For this review, take the finished solid that the model builds, in its own axes (mm). A direction names the side the tool comes from. Round coordinates to 2 decimals unless told otherwise and drop trailing zeros. Order: outer loops, then holes, each group sorted by start corner. A loop starts at its lowest first (then second) coordinate and runs counter-clockwise, first axis right, second up. Notation, with made-up numbers: (8, 17) - (61, 17) arc R23 cw to (61, 43) - close; hole circle Ø2 at (-27.5, 12.5). An arc over 180 degrees is marked (long way). One line per item, written item: value.
```python
from build123d import *

# Parameters (mm, degrees)
SKETCH1_W           = 25.4
SKETCH1_H           = 25.4
BOSS_EXTRUDE1_DEPTH = 12.7
SKETCH3_R           = 3.6576
CUT_EXTRUDE1_DEPTH  = 4.445
SKETCH2_W           = 13.97
SKETCH2_H           = 13.208
CUT_EXTRUDE2_DEPTH  = 8.255
SKETCH4_W           = 1.27
SKETCH4_H           = 6.985
CUT_EXTRUDE3_DEPTH  = 3.175
BOSS_EXTRUDE2_DEPTH = 25.4
FILLET1_R           = 3.175
SKETCH6_W           = 6.35
SKETCH6_H           = 1.5875
BOSS_EXTRUDE3_DEPTH = 6.35
BOSS_EXTRUDE4_DEPTH = 6.35
SKETCH8_R           = 0.79375
CUT_EXTRUDE4_DEPTH  = 1.5875


with BuildPart() as part:
    # Sketch1 → Boss-Extrude1 (new body)
    with BuildSketch(Plane(origin=(0, 0, 0), x_dir=(1, 0, 0), z_dir=(0, 1, 0))):
        with Locations((12.7, 12.7)):
            Rectangle(SKETCH1_W, SKETCH1_H)
    extrude(amount=BOSS_EXTRUDE1_DEPTH)

    # Sketch3 → Cut-Extrude1 (cut)
    with BuildSketch(Plane(origin=(0, 12.7, 0), x_dir=(1, 0, 0), z_dir=(0, 1, 0))):
        with Locations(Location((12.7, 12.7, 0), (0, 0, 270))):
            Circle(SKETCH3_R)
    extrude(amount=-CUT_EXTRUDE1_DEPTH, mode=Mode.SUBTRACT)

    # Sketch2 → Cut-Extrude2 (cut)
    with BuildSketch(Plane.XZ):
        with Locations((12.7, -12.7)):
            Rectangle(SKETCH2_W, SKETCH2_H)
    extrude(amount=-CUT_EXTRUDE2_DEPTH, mode=Mode.SUBTRACT)

    # Sketch4 → Cut-Extrude3 (cut)
    with BuildSketch(Plane.XZ):
        with Locations((5.08, -12.7)):
            Rectangle(SKETCH4_W, SKETCH4_H)
        with Locations((20.32, -12.7)):
            Rectangle(SKETCH4_W, SKETCH4_H)
    extrude(amount=-CUT_EXTRUDE3_DEPTH, mode=Mode.SUBTRACT)

    # Sketch5 → Boss-Extrude2 (add)
    with BuildSketch(Plane.ZY):
        Polygon((0, 0), (21.997045256, 0), (0, 12.7), align=None)
    extrude(amount=-BOSS_EXTRUDE2_DEPTH)

    # Fillet1
    fillet1_edges = [part.edges().sort_by_distance(p)[0] for p in [
        (12.7, 0, 21.997045256),
    ]]
    fillet(fillet1_edges, radius=FILLET1_R)

    # Sketch6 → Boss-Extrude3 (add)
    with BuildSketch(Plane.XZ):
        with Locations((12.7, -5.30225)):
            Rectangle(SKETCH6_W, SKETCH6_H)
        with Locations((12.7, -20.09775)):
            Rectangle(SKETCH6_W, SKETCH6_H)
    extrude(amount=BOSS_EXTRUDE3_DEPTH)

    # Sketch7 → Boss-Extrude4 (add)
    with BuildSketch(Plane.ZY.offset(-9.525)):
        Polygon((-4.5085, -6.35), (-1.547446371, 0), (-4.5085, 0), align=None)
        Polygon((-20.8915, -6.35), (-23.852553629, 0), (-20.8915, 0), align=None)
    extrude(amount=-BOSS_EXTRUDE4_DEPTH)

    # Sketch8 → Cut-Extrude4 (cut, symmetric)
    with BuildSketch(Plane.ZY.offset(-12.7)):
        with Locations((-19.304, -3.27025)):
            Circle(SKETCH8_R)
        with Locations((-6.096, -3.27025)):
            Circle(SKETCH8_R)
    extrude(amount=CUT_EXTRUDE4_DEPTH, both=True, mode=Mode.SUBTRACT)


solid = part.part
```
Item 1: Take a section at D-D (x = 7.75). Write out the cut boundary in (y, z) (3 decimals).
Returned:
outline: (0, -25.4) - (12.7, -25.4) - (12.7, 0) - (5.925, 11.735) arc R3.175 ccw to (0, 10.148) - (0, -6.096) - (8.255, -6.096) - (8.255, -19.304) - (0, -19.304) - close
Item 2: For P1, Ø2.5, axis at y = -3.5, z = -3, coming from the +X side (3 decimals); P2, Ø7, axis at x = 9.5, y = -1.5, coming from the +Z side; P3, Ø1.5, axis at x = 16.5, z = -12.5, coming from the -Y side (3 decimals), all flat-tipped, find the tip position at first contact; note any pin that passes through.
Returned:
P1: x = 15.875
P2: z = 13.1
P3: y = 8.255
Item 3: Wall thickness on line 1 (X direction, y = 11.7, z = -12.7); line 2 (X direction, y = 5.25, z = -10) (3 decimals); line 3 (Y direction, x = 6.25, z = 5.5): over which ranges is each line inside the solid? List them lowest first.
Returned:
line 1: 0 to 9.04, 16.36 to 25.4
line 2: 0 to 5.715, 19.685 to 25.4
line 3: 0 to 9.52
Item 4: The part is to be moulded in two halves that separate along X. For faces 4 (the flat face through (5, 3.175, -13)), 5 (the flat face through (9.525, -2, -4)), 6 (the flat face through (15.875, -2, -4)), say which applies: +X half, -X half, draft (parallel to the pull), parting line (faces both ways), or undercut.
Returned:
face 4: undercut
face 5: -X half
face 6: +X half
Item 5: Take a section at A-A (z = -12.7). Write out the cut boundary in (x, y) (3 decimals).
Returned:
outline: (0, 0) - (4.445, 0) - (4.445, 3.175) - (5.715, 3.175) - (5.715, 8.255) - (9.042, 8.255) - (9.042, 12.7) - (0, 12.7) - close; (16.358, 8.255) - (19.685, 8.255) - (19.685, 3.175) - (20.955, 3.175) - (20.955, 0) - (25.4, 0) - (25.4, 12.7) - (16.358, 12.7) - close
Item 6: Machinability: for faces 1 (the flat face through (20, 2, -16.192)), 2 (the flat face through (25.4, 6, -6)), 3 (the cylindrical face through (12.678, -3.288, -5.302)), which of the approach directions +Z, -Z, +X, -X, +Y, -Y give a long, thin tool a straight path to every point of the face, cutting with its end or side? Answer none if there is none.
Returned:
face 1: -Y
face 2: +Z, -Z, +X, +Y, -Y
face 3: none
Item 7: Take a section at C-C (y = -4.5). Write out the cut boundary in (x, z) (3 decimals), plus the area to 3 significant figures.
Returned:
outline: (9.525, -21.754) - (15.875, -21.754) - (15.875, -19.304) - (9.525, -19.304) - close; (9.525, -6.096) - (15.875, -6.096) - (15.875, -3.646) - (9.525, -3.646) - close
area: 31.1 mm^2
